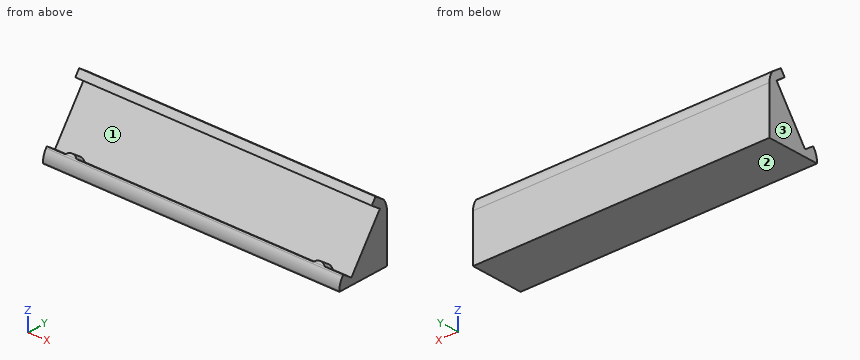
from build123d import *

# Parameters (mm, degrees)
F1_DEPTH    = 40
F2_R        = 5
F3_T1_DEPTH = 95
F5_DEPTH    = 3


# Not quite as in the source:
# - a fillet or chamfer that OpenCascade refuses, or shapes differently, is made with other operations: its cross-section is extruded or revolved along the edge and cut away or added


with BuildPart() as f1:
    # F0 (on Right) → F1 (new body, symmetric)
    with BuildSketch(Plane.YZ):
        Polygon((0.0953060592, 0.1361111585), (0, 0), (11.9932583499, 0), (11.9932583499, 15.7), (10.9932583499, 15.7), (9.8461054772, 14.0616959114), (1.2424589319, 1.7744152471), align=None)
        Polygon((7.3886493443, 15.7824252205), (9.8461054772, 14.0616959114), (10.9932583499, 15.7), (8.535802217, 17.4207293091), align=None)
        Polygon((-2.3621500736, 1.8568404676), (0.0953060592, 0.1361111585), (1.2424589319, 1.7744152471), (-1.2149972009, 3.4951445561), align=None)
        Polygon((-2.3621500736, 0), (0, 0), (0.0953060592, 0.1361111585), (-2.3621500736, 1.8568404676), align=None)
    extrude(amount=F1_DEPTH, both=True)

    # F2
    f2_edges = [f1.edges().sort_by_distance(p)[0] for p in [
        (0, -2.36215, 1.85684),
    ]]
    fillet(f2_edges, radius=F2_R)

    # F3: fillet of radius 5 on 1 edges, made by hand

    # F3_s2 → F3_t1 (cut)
    with BuildSketch(Plane.YZ.offset(-47.5)):
        with BuildLine():
            ThreePointArc((11.9932583499, 12.7), (11.7366748401, 14.2811388301), (10.9932583499, 15.7))
            Line((10.9932583499, 15.7), (11.9932583499, 15.7))
            Line((11.9932583499, 15.7), (11.9932583499, 12.7))
        make_face()
    extrude(amount=F3_T1_DEPTH, mode=Mode.SUBTRACT)

    # F4 (on face) → F5 (join)
    with BuildSketch(Plane(origin=(0, 0, 0), x_dir=(1, 0, 0), z_dir=(0, -0.8191520443, 0.5735764364))):
        with BuildLine():
            Line((-35, 2.1661610436), (-32, 2.1661610436))
            ThreePointArc((-32, 2.1661610436), (-33.5, 2.843285388), (-35, 2.1661610436))
        make_face()
        with BuildLine():
            ThreePointArc((35, 2.1661610436), (33.5, 2.843285388), (32, 2.1661610436))
            Line((32, 2.1661610436), (35, 2.1661610436))
        make_face()
    extrude(amount=F5_DEPTH)


solid = f1.part
Source: CAD feature listing. Evaluate the final solid. Frame: model axes, mm. Face numbers are marked on the shaded views. Give positions to 0.01 mm unless a question says otherwise; leave off trailing zeros. Loops run counter-clockwise (first coordinate to the right, second up) from the corner with the lowest first, then second, coordinate; pieces in that order, holes last. Notation, with made-up numbers: (37, 29) -> (62, 29) arc R18 cw to (62, 58) -> close; hole circle Ø2 at (-12.5, 67). An arc over 180 degrees is marked (long way). Use a Markdown table: item, result. Add a question column.
1) Section query A-A, the plane x = 0. Return the cut outline in (y, z) (3 decimals), then the cut area to 3 significant figures.
2) Section query B-B, the plane z = 6. Return the cut outline in (x, y).
3) Line query: line 1 along Z through (x, y) = (-14, 8.5); line 2 along Y through (x, z) = (18, 2); line 3 along Z through (x, y) = (-15.5, -0.75). Output: solid intervals per line, ascending. Write a range as [from, to].
4) Pull-direction query (Z, two-part tool) for the marked faces 1, 2 and 3; classes: +Z half, -Z half, draft (parallel to the pull), parting line (faces both ways), or undercut.
5) Section query C-C, the plane y = 3.5. Return the cut outline in (x, z), then the cut area to 3 significant figures.
6) First-contact query: pin 1 (1 mm diameter, centred on x = 12.5, y = 1, fed in from +Z); pin 2 (1.5 mm diameter, centred on x = -3, y = 7, fed in from +Z); pin 3 (6 mm diameter, centred on y = 1.5, z = 11.5, fed in from -X). Flat tips, straight axial feed; report the tip coordinate or a pass-through.
Numbers:
| question | item | result |
|---|---|---|
| 1 | outline | (-2.362, 0) -> (11.993, 0) -> (11.993, 12.7) arc R5 ccw to (10.993, 15.7) -> (8.536, 17.421) -> (7.389, 15.782) -> (9.846, 14.062) -> (1.242, 1.774) -> (-1.215, 3.495) -> (-1.458, 3.148) arc R5 ccw to (-2.362, 0.28) -> close |
| 1 | area | 115 mm2 |
| 2 | outline | (-40, 4.2) -> (40, 4.2) -> (40, 11.99) -> (-40, 11.99) -> close |
| 3 | line 1 | z = [0, 12.14], [15, 17.37] |
| 3 | line 2 | y = [-2.06, 0.92], [1.4, 11.99] |
| 3 | line 3 | z = [0, 3.17] |
| 4 | face 1 | undercut |
| 4 | face 2 | -Z half |
| 4 | face 3 | draft |
| 5 | outline | (-40, 0) -> (40, 0) -> (40, 5) -> (-40, 5) -> close |
| 5 | area | 400 mm2 |
| 6 | pin 1 | stops at z = 2.29 |
| 6 | pin 2 | stops at z = 16.3 |
| 6 | pin 3 | passes through |
